For this review, take the finished solid that the model builds, in its own axes (mm). Face numbers are marked on the shaded views. A direction names the side the tool comes from. Round coordinates to 2 decimals unless told otherwise and drop trailing zeros. Loops run counter-clockwise (first coordinate to the right, second up) from the corner with the lowest first, then second, coordinate; pieces in that order, holes last.
1) Tool access review of the marked faces 1, 2 and 3: name each direction out of +Z, -Z, +X, -X, +Y, -Y from which nothing blocks a thin tool from reaching the whole face with its end or side.
2) Take a section at A-A (x = 0). State the section outline as (y, z) points.
3) Wall thickness on L1, parallel to Z at x = -2, y = -10; L2, parallel to Z at x = 6, y = 11.5; L3, parallel to X at y = -2, z = 0: over which ranges is each line inside the solid? List them lowest first.
4) Take a section at C-C (y = 11). State the section outline as (x, z) points.
5) Take a section at B-B (z = 0). State the section outline as (x, y) points, then the cut area to 3 significant figures.
6) Mouldability with a two-part tool opening along X and no side actions: class the marked faces 4, 5, 6 and 7 as pulls with the +X half, pulls with the -X half, needs draft (parallel to the pull), parting line crosses it, or undercut.
7) Insertion check: pin 1 (6 mm diameter, centred on x = 2, y = 11, fed in from -Z); pin 2 (4 mm diameter, centred on x = -32, z = -18.5, fed in from -Y); pin 3 (4 mm diameter, centred on x = -28, y = -10.5, fed in from -Z). Each pin has a flat end and moves straight along its axis. Give the tip position at first contact, or say it passes through.
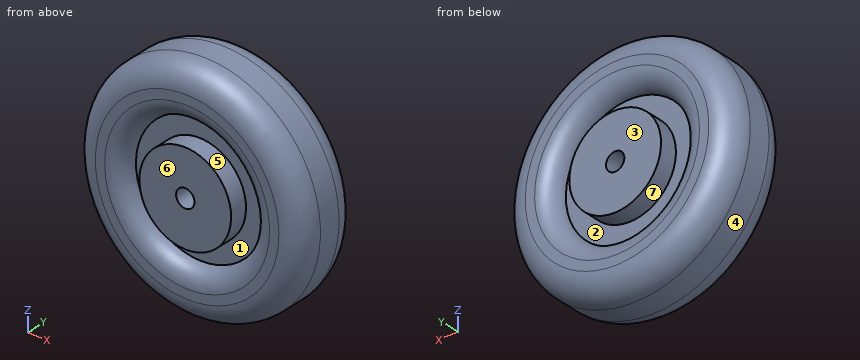
```python
from build123d import *

# Parameters (mm, degrees)
CONG_1_R = 10
CONG_2_R = 8


with BuildPart() as part:
    # Esquisse1 → Révolution1 (revolve)
    with BuildSketch(Plane.XY, mode=Mode.PRIVATE) as r_volution1_sk:
        Polygon((-4, -16), (-4, 16), (-20, 16), (-20, 8), (-28, 8), (-28, 15), (-50, 15), (-50, -15), (-28, -15), (-28, -8), (-20, -8), (-20, -16), align=None)
    revolve(r_volution1_sk.sketch.rotate(Axis((0, 0, 0), (0, 1, 0)), 270), axis=Axis((0, 0, 0), (0, 1, 0)))

    # Congé1
    cong_1_edges = [part.edges().sort_by_distance(p)[0] for p in [
        (0, -15, 50),
        (0, 15, 50),
    ]]
    fillet(cong_1_edges, radius=CONG_1_R)

    # Congé2
    # the kernel refuses this fillet: 8 mm, written as the material it takes off along each edge
    with BuildSketch(Plane(origin=(0, -15, 0), x_dir=(0, 0, -1), z_dir=(1, 0, 0))) as cong_2_piece_1:
        with BuildLine():
            CenterArc((35.937253933, 8), CONG_2_R, 187.180755781, 82.819244219)
            Line((28, 7), (27.841254921, 6.98))
            ThreePointArc((27.841254921, 6.98), (27.84, 3.5), (27.84, 0))
            Line((27.84, 0), (28, -0.16))
            Line((28, -0.16), (35.937253933, -0.16))
            Line((35.937253933, -0.16), (35.937253933, 0))
        make_face()
    revolve(axis=Axis((0, -15, 0), (0, 1, 0)), mode=Mode.SUBTRACT)
    with BuildSketch(Plane(origin=(0, 15, 0), x_dir=(0, 0, -1), z_dir=(1, 0, 0))) as cong_2_piece_2:
        with BuildLine():
            CenterArc((35.937253933, -8), CONG_2_R, 90, 82.819244219)
            Line((28, -7), (27.841254921, -6.98))
            ThreePointArc((27.841254921, -6.98), (27.84, -3.5), (27.84, 0))
            Line((27.84, 0), (28, 0.16))
            Line((28, 0.16), (35.937253933, 0.16))
            Line((35.937253933, 0.16), (35.937253933, 0))
        make_face()
    revolve(axis=Axis((0, 15, 0), (0, 1, 0)), mode=Mode.SUBTRACT)


solid = part.part
```
Response:
1. face 1: -Y
1. face 2: +Y
1. face 3: +Z, -Z, +X, -X, +Y
2. outline: (-16, -20) - (-8, -20) - (-8, -28) arc R8 ccw to (-15, -35.94) - (-15, -40) arc R10 ccw to (-5, -50) - (5, -50) arc R10 ccw to (15, -40) - (15, -35.94) arc R8 ccw to (8, -28) - (8, -20) - (16, -20) - (16, -4) - (-16, -4) - close; (-16, 4) - (16, 4) - (16, 20) - (8, 20) - (8, 28) arc R8 ccw to (15, 35.94) - (15, 40) arc R10 ccw to (5, 50) - (-5, 50) arc R10 ccw to (-15, 40) - (-15, 35.94) arc R8 ccw to (-8, 28) - (-8, 20) - (-16, 20) - close
3. L1: z = -48.62 to -28.45, -19.9 to -3.46, 3.46 to 19.9, 28.45 to 48.62
3. L2: z = -47.22 to -28.7, -19.08 to 19.08, 28.7 to 47.22
3. L3: x = -50 to -4, 4 to 50
4. outline: circle Ø96 at (0, 0); circle Ø40 at (0, 0); hole circle Ø58.02 at (0, 0); hole circle Ø8 at (0, 0)
5. outline: (-50, -5) arc R10 ccw to (-40, -15) - (-35.94, -15) arc R8 ccw to (-28, -8) - (-20, -8) - (-20, -16) - (-4, -16) - (-4, 16) - (-20, 16) - (-20, 8) - (-28, 8) arc R8 ccw to (-35.94, 15) - (-40, 15) arc R10 ccw to (-50, 5) - close; (4, -16) - (20, -16) - (20, -8) - (28, -8) arc R8 ccw to (35.94, -15) - (40, -15) arc R10 ccw to (50, -5) - (50, 5) arc R10 ccw to (40, 15) - (35.94, 15) arc R8 ccw to (28, 8) - (20, 8) - (20, 16) - (4, 16) - close
5. area: 2,460 mm2
6. face 4: parting line crosses it
6. face 5: undercut
6. face 6: needs draft
6. face 7: undercut
7. pin 1: stops at z = -49.51
7. pin 2: stops at y = -15
7. pin 3: stops at z = -41.32
